```python
from build123d import *

# Parameters (mm, degrees)
SKETCH1_R                = 25
BOSS_EXTRUDE1_DEPTH      = 10
BOSS_EXTRUDE3_START      = -10
SKETCH2_W                = 5
SKETCH2_H                = 59.633486872
BOSS_EXTRUDE3_DEPTH      = 10
SKETCH3_R                = 3
CUT_EXTRUDE1_DEPTH       = 29
FILLET1_R                = 5
CIRPATTERN1_COUNT        = 3
FILLET1_OF_CIRPATTERN1_R = 5
BOSS_EXTRUDE5_START      = 5
SKETCH5_R                = 25
SKETCH5_R_2              = 22.5
BOSS_EXTRUDE5_DEPTH      = 5


with BuildPart() as part:
    # Sketch1 → Boss-Extrude1 (new body)
    with BuildSketch(Plane.XY):
        Circle(SKETCH1_R)
        with BuildLine():
            Line((-2.5, 12.5), (2.5, 12.5))
            ThreePointArc((2.5, 12.5), (9.571067812, 9.571067812), (12.5, 2.5))
            Line((12.5, 2.5), (12.5, -2.5))
            ThreePointArc((12.5, -2.5), (9.571067812, -9.571067812), (2.5, -12.5))
            Line((2.5, -12.5), (-2.5, -12.5))
            ThreePointArc((-2.5, -12.5), (-9.571067812, -9.571067812), (-12.5, -2.5))
            Line((-12.5, -2.5), (-12.5, 2.5))
            ThreePointArc((-12.5, 2.5), (-9.571067812, 9.571067812), (-2.5, 12.5))
        make_face(mode=Mode.SUBTRACT)
    extrude(amount=BOSS_EXTRUDE1_DEPTH)

    # Sketch2 → Boss-Extrude3 (add)
    with BuildSketch(Plane.XY.offset(10).offset(BOSS_EXTRUDE3_START)):
        with BuildLine():
            Line((-7.5, 81.5), (-12.5, 81.5))
            Line((-12.5, 81.5), (-12.5, 21.650635095))
            ThreePointArc((-12.5, 21.650635095), (-10.060200326, 22.886510643), (-7.5, 23.848480035))
            Line((-7.5, 23.848480035), (-7.5, 81.5))
        make_face()
        with Locations((10, 51.683256564)):
            Rectangle(SKETCH2_W, SKETCH2_H)
    boss_extrude3 = extrude(amount=BOSS_EXTRUDE3_DEPTH)

    # Sketch3 → Cut-Extrude1 (cut)
    with BuildSketch(Plane(origin=(12.5, 0, 0), x_dir=(0, 0, -1), z_dir=(1, 0, 0))):
        with Locations((-5, 71.5)):
            Circle(SKETCH3_R)
    cut_extrude1 = extrude(amount=-CUT_EXTRUDE1_DEPTH, mode=Mode.SUBTRACT)

    # Fillet1
    fillet1_edges = [part.edges().sort_by_distance(p)[0] for p in [
        (-10, 81.5, 10),
        (-10, 81.5, 0),
        (10, 81.5, 10),
        (10, 81.5, 0),
    ]]
    fillet(fillet1_edges, radius=FILLET1_R - 0.0001)  # a hair under: the kernel refuses the full size

    # CirPattern1: Boss-Extrude3, Cut-Extrude1 ×3 about axis
    cirpattern1_axis = Axis((0, 0, 0), (0, 0, 1))
    add([boss_extrude3.rotate(cirpattern1_axis, i * 360 / CIRPATTERN1_COUNT) for i in range(1, CIRPATTERN1_COUNT)])
    add([cut_extrude1.rotate(cirpattern1_axis, i * 360 / CIRPATTERN1_COUNT) for i in range(1, CIRPATTERN1_COUNT)], mode=Mode.SUBTRACT)

    # Fillet1 of CirPattern1
    fillet1_of_cirpattern1_edges = [part.edges().sort_by_distance(p)[0] for p in [
        (-65.581070408, -49.410254038, 10),
        (-65.581070408, -49.410254038, 0),
        (-75.581070408, -32.089745962, 10),
        (-75.581070408, -32.089745962, 0),
        (75.581070408, -32.089745962, 10),
        (75.581070408, -32.089745962, 0),
        (65.581070408, -49.410254038, 10),
        (65.581070408, -49.410254038, 0),
    ]]
    fillet(fillet1_of_cirpattern1_edges, radius=FILLET1_OF_CIRPATTERN1_R - 0.0001)  # a hair under: the kernel refuses the full size

    # Sketch5 → Boss-Extrude5 (add)
    with BuildSketch(Plane(origin=(0, 0, 0), x_dir=(-1, 0, 0), z_dir=(0, 0, -1)).offset(BOSS_EXTRUDE5_START)):
        Circle(SKETCH5_R)
        Circle(SKETCH5_R_2, mode=Mode.SUBTRACT)
    extrude(amount=-BOSS_EXTRUDE5_DEPTH)


solid = part.part
```
Geometry check sheet. Reference: the model listing, model coordinates, mm. A direction names the side the tool comes from. Give positions to 0.01 mm unless a question says otherwise; leave off trailing zeros. Loops run counter-clockwise (first coordinate to the right, second up) from the corner with the lowest first, then second, coordinate; pieces in that order, holes last. Notation, with made-up numbers: (39.5, 57) - (71.5, 57) arc R29 ccw to (71.5, 93) - close; hole circle Ø7 at (58, 19). An arc over 180 degrees is marked (long way). Use CSV: the item, a comma, the result in double quotes. Start each with the question number.
Q1. Scan lines: probe 1 along X at (y, z) = (37, 6.5); probe 2 along Y at (x, z) = (0, -1.7); probe 3 along X at (y, z) = (-6, 0.25). Record each from-to range of solid material in increasing order. Write a range as from..to.
Q2. Access from +Z, -Z, +X, -X, +Y, -Y to the whole of each face (thin tool, end or side, straight path). Record for faces 4 (the face through (-38.778, -36.822, 4.93)), 5 (the face through (7.5, 52, 5)), 6 (the face through (0, -12.5, 5)), 7 (the face through (64.329, -48.728, 8.496)), 8 (the face through (37, -33, 0)).
Q3. Section check D-D, the plane x = -43. Record the cut outline in (y, z).
Q4. Section check C-C, the plane y = 71.5. Record the cut outline in (x, z), and give its area (3 significant figures).
Q5. Section check B-B, the plane x = 0. Record the cut outline in (y, z).
Q6. Release check for a two-part mould opening along X. For faces 1 (the face through (-10, 49, 0)), 2 (the face through (-12.5, 52, 5)), 3 (the face through (9.49, 9.65, 4.93)) record: +X half, -X half, draft (parallel to the pull), parting line (faces both ways), or undercut.
Q7. Section check A-A, the plane y = 54. Record the cut outline in (x, z), and give its area (3 significant figures).
Q8. Go/stop test with flat-tipped pins: pin 1 Ø5.5 at (x, z) = (-0.5, 7) entering from -Y; pin 2 Ø4 at (x, z) = (1, 5) entering from +Y; pin 3 Ø5.5 at (y, z) = (71.5, 5) entering from +X; pin 4 Ø8 at (x, z) = (-51.5, -3) entering from -Y. Record where each tip stops, or that it passes through.
Findings below:
1,probe 1,"x = -12.5..-7.5, 7.5..12.5"
1,probe 2,"y = -25..-22.5, 22.5..25"
1,probe 3,"x = -35.39..-25.39, -24.27..-11.87, 11.87..24.27, 25.39..35.39"
2,face 4,"+Z, -Z, -Y"
2,face 5,"+Z, -Z, +Y"
2,face 6,"+Z, -Z"
2,face 7,"+Z, +X, -Y"
2,face 8,"-Z, +X, -Y"
3,outline,"(-39.26, 0) - (-33.49, 0) - (-33.49, 10) - (-39.26, 10) - close; (-16.17, 0) - (-10.39, 0) - (-10.39, 10) - (-16.17, 10) - close"
4,outline,"(-12.5, 0) - (-7.5, 0) - (-7.5, 2) - (-12.5, 2) - close; (-12.5, 8) - (-7.5, 8) - (-7.5, 10) - (-12.5, 10) - close; (7.5, 0) - (12.5, 0) - (12.5, 2) - (7.5, 2) - close; (7.5, 8) - (12.5, 8) - (12.5, 10) - (7.5, 10) - close"
4,area,"40.0 mm^2"
5,outline,"(-25, -5) - (-22.5, -5) - (-22.5, 0) - (-12.5, 0) - (-12.5, 10) - (-25, 10) - close; (12.5, 0) - (22.5, 0) - (22.5, -5) - (25, -5) - (25, 10) - (12.5, 10) - close"
6,face 1,"draft"
6,face 2,"-X half"
6,face 3,"undercut"
7,outline,"(-12.5, 0) - (-7.5, 0) - (-7.5, 10) - (-12.5, 10) - close; (7.5, 0) - (12.5, 0) - (12.5, 10) - (7.5, 10) - close"
7,area,"100 mm^2"
8,pin 1,"stops at y = -25"
8,pin 2,"stops at y = 25"
8,pin 3,"passes through"
8,pin 4,"stops at y = -45.69"
